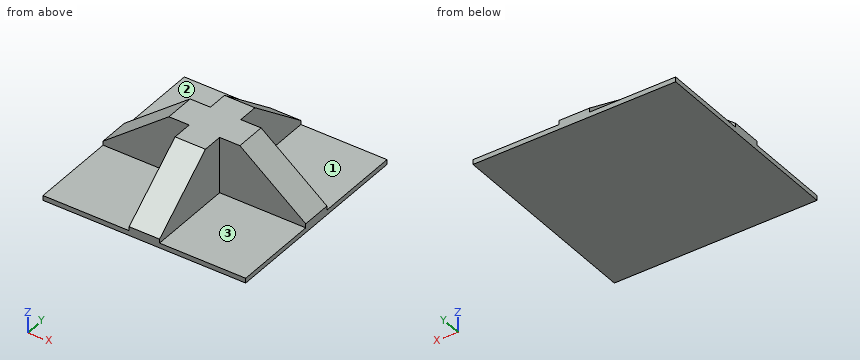
Autodesk Inventor part; units mm, degrees
ref_plane "YZ Plane" through (0, 0, 0) normal (1, 0, 0) x (0, 1, 0)
ref_plane "XZ Plane" through (0, 0, 0) normal (0, 1, 0) x (-1, 0, 0)
ref_plane "XY Plane" through (0, 0, 0) normal (0, 0, 1) x (1, 0, 0)
sketch "スケッチ1" plane through (0, 0, 0) normal (0, 0, 1) x (1, 0, 0)
  line L0 (250, 250) -> (250, -250)
  line L1 (250, -250) -> (-250, -250)
  line L2 (-250, -250) -> (-250, 250)
  line L3 (-250, 250) -> (250, 250)
  point P0 (0, 0)
  point P1 (0, 0)
  dimension "d0" = 500
extrude "押し出し1" add sketch "スケッチ1" along normal blind 12
sketch "スケッチ2" plane through (0, 0, 12) normal (0, 0, 1) x (1, 0, 0)
  line L0 (250, -250) -> (250, 250)
  line L1 (250, 250) -> (-250, 250)
  line L2 (-250, 250) -> (-250, -250)
  line L3 (-250, -250) -> (250, -250)
  line L4 (-250, -250) -> (-37.5, -250)
  line L5 (-250, -250) -> (250, -250)
  line L6 (-37.5, -250) -> (37.5, -250)
  line L7 (-37.5, -250) -> (-37.5, 250)
  line L8 (37.5, -250) -> (37.5, 250)
  line L9 (250, 250) -> (-250, 250)
  line L10 (-250, -250) -> (-250, -37.5)
  line L11 (-250, 250) -> (-250, -250)
  line L12 (-250, -37.5) -> (250, -37.5)
  line L13 (-250, -37.5) -> (-250, 37.5)
  line L14 (-250, 37.5) -> (250, 37.5)
  point P0 (0, 0)
  dimension "d3" = 212.5
  dimension "d4" = 75
  dimension "d5" = 212.5
  dimension "d6" = 75
extrude "押し出し2" add sketch "スケッチ2" along normal blind 10 contours L12 L8 L14 L0 | L3 L7 L12 L8 | L12 L7 L14 L8 | L14 L7 L1 L8 | L12 L2 L14 L7
sketch "スケッチ3" plane through (0, 0, 22) normal (0, 0, 1) x (1, 0, 0)
  line L0 (-37.5, -37.5) -> (-37.5, -250)
  line L1 (-37.5, -250) -> (37.5, -250)
  line L2 (37.5, -250) -> (37.5, -37.5)
  line L3 (37.5, -37.5) -> (250, -37.5)
  line L4 (250, -37.5) -> (250, 37.5)
  line L5 (250, 37.5) -> (37.5, 37.5)
  line L6 (37.5, 37.5) -> (37.5, 250)
  line L7 (37.5, 250) -> (-37.5, 250)
  line L8 (-37.5, 250) -> (-37.5, 37.5)
  line L9 (-37.5, 37.5) -> (-250, 37.5)
  line L10 (-250, 37.5) -> (-250, -37.5)
  line L11 (-250, -37.5) -> (-37.5, -37.5)
  point P0 (0, 0)
extrude "押し出し3" add sketch "スケッチ3" along normal blind 128
chamfer "面取り1" distance 162.5 distance2 128 1 edges at (-250, 0, 150) measured on face at (12.5, 179.1667, 150)
chamfer "面取り2" distance 162.5 distance2 128 1 edges at (0, -250, 150) measured on face at (12.5, 179.1667, 150)
chamfer "面取り3" distance 162.5 distance2 128 1 edges at (0, 250, 150) measured on face at (12.5, 108.3333, 150)
chamfer "面取り4" distance 162.5 distance2 128 1 edges at (250, 0, 150) measured on face at (108.3333, -12.5, 150)
sketch "スケッチ4" plane through (0, 0, 150) normal (0, 0, 1) x (1, 0, 0)
  circle A0 centre (0, 0) radius 0.005
  dimension "d23" = 0.01
extrude "押し出し4" cut sketch "スケッチ4" against normal through all
properties part number "障害物、山"
The listing builds one solid part. Answer for the finished solid, in the listing's coordinates (mm). Face numbers are marked on the shaded views. A direction names the side the tool comes from. Coordinates: 2 decimals unless noted, no trailing zeros. Loops run counter-clockwise (first coordinate to the right, second up) from the corner with the lowest first, then second, coordinate; pieces in that order, holes last. Notation, with made-up numbers: (1, -7.5) - (30, -7.5) arc R20 ccw to (30, 24.5) - close; hole circle Ø5 at (-23.75, 70.5). An arc over 180 degrees is marked (long way). Use a Markdown table: item, result. Add a question column.
1) The part is cut by section C-C, the plane y = 114. Give the vertices of the cut face in (x, z).
2) Find the intervals of material crossed by line 1 (X direction, y = -49.5, z = 51); line 2 (Z direction, x = -169, y = -68), in increasing order.
3) Given pin 1 (3 mm diameter, centred on x = 191, y = -52.5, fed in from -Z); pin 2 (1 mm diameter, centred on y = 18, z = 100.5, fed in from +X); pin 3 (8 mm diameter, centred on y = 110.5, z = 130, fed in from +X); pin 4 (3 mm diameter, centred on x = -123, z = 80, fed in from -Y), each flat-ended and moving along its own axis, determine where each tip first touches the part or whether it passes through.
4) For the marked faces 1, 2 and 3, determine the directions among +Z, -Z, +X, -X, +Y, -Y from which every point of the face is accessible in a straight line to the end or side of a thin tool.
5) The part is cut by section A-A, the plane x = 74.5. Give the vertices of the cut face in (y, z).
6) The part is cut by section D-D, the plane x = -23.5. Give the vertices of the cut face in (y, z), and give its area (3 significant figures).
Here are the results:
| question | item | result |
|---|---|---|
| 1 | outline | (-250, 0) - (250, 0) - (250, 12) - (37.5, 12) - (37.5, 129.13) - (-37.5, 129.13) - (-37.5, 12) - (-250, 12) - close |
| 2 | line 1 | x = -37.5 to 37.5 |
| 2 | line 2 | z = 0 to 12 |
| 3 | pin 1 | stops at z = 0 |
| 3 | pin 2 | stops at x = 150.98 |
| 3 | pin 3 | stops at x = 37.5 |
| 3 | pin 4 | stops at y = -37.5 |
| 4 | face 1 | +Z, +X, +Y |
| 4 | face 2 | +Z, -X, +Y |
| 4 | face 3 | +Z, +X, -Y |
| 5 | outline | (-250, 0) - (250, 0) - (250, 12) - (37.5, 12) - (37.5, 150) - (-37.5, 150) - (-37.5, 12) - (-250, 12) - close |
| 6 | outline | (-250, 0) - (250, 0) - (250, 22) - (87.5, 150) - (-87.5, 150) - (-250, 22) - close |
| 6 | area | 54,200 mm^2 |
